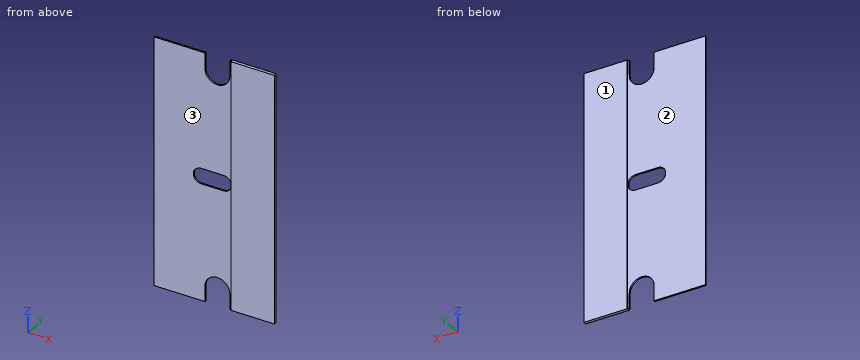
from build123d import *

# Parameters (mm, degrees)
F1_DEPTH      = 40.64
F3_DEPTH      = 0.255
F3_DEPTH_BACK = 0.255


with BuildPart() as f1:
    # F0 (on Top) → F1 (new body)
    with BuildSketch(Plane.XY):
        Polygon((0, 0.127), (-12.7, 0.127), (-12.7, -0.127), (0, -0.127), (0, -0.254), (7.112, -0.254), (7.112, 0.254), (0, 0.254), align=None)
    extrude(amount=F1_DEPTH)

    # F2 (on Front) → F3 (cut, two sides)
    with BuildSketch(Plane.XZ) as f3_sk:
        with BuildLine():
            Line((-4.318, 40.64), (-4.318, 38.1))
            ThreePointArc((-4.318, 38.1), (-2.286, 36.068), (-0.254, 38.1))
            Line((-0.254, 38.1), (-0.254, 40.64))
            Line((-0.254, 40.64), (-4.318, 40.64))
        make_face()
        with BuildLine():
            Line((-4.318, 2.54), (-4.318, 0))
            Line((-4.318, 0), (-0.254, 0))
            Line((-0.254, 0), (-0.254, 2.54))
            ThreePointArc((-0.254, 2.54), (-2.286, 4.572), (-4.318, 2.54))
        make_face()
        with BuildLine():
            Line((-1.27, 21.59), (-4.953, 21.59))
            ThreePointArc((-4.953, 21.59), (-6.223, 20.32), (-4.953, 19.05))
            Line((-4.953, 19.05), (-1.27, 19.05))
            ThreePointArc((-1.27, 19.05), (0, 20.32), (-1.27, 21.59))
        make_face()
    extrude(amount=-F3_DEPTH, mode=Mode.SUBTRACT)
    extrude(f3_sk.sketch, amount=F3_DEPTH_BACK, mode=Mode.SUBTRACT)


solid = f1.part
CAD build for the part. Positions are in the model's coordinates, mm. Face numbers are marked on the shaded views. A direction names the side the tool comes from. Give positions to 0.01 mm unless a question says otherwise; leave off trailing zeros. Loops run counter-clockwise (first coordinate to the right, second up) from the corner with the lowest first, then second, coordinate; pieces in that order, holes last. Notation, with made-up numbers: M 51.5,67.5 L 108.5,67.5 A23 cw 108.5,103.5 Z; hole C -34.5,24.25 d10. An arc over 180 degrees is marked long. Answer in a Markdown table with one row per item. Add a question column.
Item 1: Probe probe 1 along Y at (x, z) = (-8.5, 29.5); probe 2 along X at (y, z) = (-0.2, 16.5); probe 3 along X at (y, z) = (0, 20). List the from-to ranges inside material, lowest first.
Item 2: Band-saw the part on A-A on y = 0. Give the cut face in (x, z).
Item 3: Tool access for the marked faces 1, 2 and 3: list every direction of +Z, -Z, +X, -X, +Y, -Y with a clear straight run to the whole face (end or side of a thin tool).
Item 4: Drop flat-ended pins along their axis: P1, Ø1, axis at x = -5, z = 10.5, coming from the -Y side; P2, Ø4, axis at x = -9, z = 25.5, coming from the +Y side. Give the stop position or say it passes through.
Item 5: Band-saw the part on B-B on z = 7.5. Give the cut face in (x, y), then the cut area to 3 significant figures.
Item 6: Band-saw the part on C-C on x = -10. Give the cut face in (y, z).
Reply:
| question | item | result |
|---|---|---|
| 1 | probe 1 | y = -0.13 to 0.13 |
| 1 | probe 2 | x = 0 to 7.11 |
| 1 | probe 3 | x = -12.7 to -6.18, -0.04 to 7.11 |
| 2 | outline | M -12.7,0 L -4.32,0 L -4.32,2.54 A2.03 cw -0.25,2.54 L -0.25,0 L 7.11,0 L 7.11,40.64 L -0.25,40.64 L -0.25,38.1 A2.03 cw -4.32,38.1 L -4.32,40.64 L -12.7,40.64 Z; hole M -4.95,19.05 L -1.27,19.05 A1.27 ccw -1.27,21.59 L -4.95,21.59 A1.27 ccw Z |
| 3 | face 1 | +Z, -Z, +X, -X, +Y |
| 3 | face 2 | +Z, -Z, -X, +Y |
| 3 | face 3 | +Z, -Z, -X, -Y |
| 4 | P1 | stops at y = -0.13 |
| 4 | P2 | stops at y = 0.13 |
| 5 | outline | M -12.7,-0.13 L 0,-0.13 L 0,-0.25 L 7.11,-0.25 L 7.11,0.25 L 0,0.25 L 0,0.13 L -12.7,0.13 Z |
| 5 | area | 6.84 mm^2 |
| 6 | outline | M -0.13,0 L 0.13,0 L 0.13,40.64 L -0.13,40.64 Z |
